Part model, mm, in its own coordinate system. A direction names the side the tool comes from. Coordinates: 2 decimals unless noted, no trailing zeros. Write each loop counter-clockwise with the first axis right and the second up, starting at its lowest first coordinate (ties: lowest second). Pieces come first, ordered by that corner, then holes. Notation, with made-up numbers: (-2.75, 31.5) -> (51.25, 31.5) arc R35 cw to (51.25, 64.5) -> close; hole circle Ø8 at (28.5, -21). An arc over 180 degrees is marked (long way). One line per question, with ' | ' between items. Start each with the question number.
Item 1: Saw through at B-B (y = 0.5). List the corners of the cut face in (x, z), and give its area (3 significant figures).
Item 2: Saw through at C-C (x = -6.25). List the corners of the cut face in (y, z), and give its area (3 significant figures).
Item 3: 3-axis set-ups, long thin cutter, end or side, ignore diameter. For faces 1 (the flat face through (4.7, 0, 14)), 2 (the flat face through (13.178, 0, -8)), 3 (the flat face through (-4.7, 0, 28)), 4 (the flat face through (3, 0, 32)): which of +Z, -Z, +X, -X, +Y, -Y reach the whole face in a straight line?
Item 4: Pin check, flat tips, straight feed: pin 1 (2.5 mm diameter, centred on x = -10.5, y = 1, fed in from +Z); pin 2 (3 mm diameter, centred on y = 2.5, z = 35.5, fed in from -X); pin 3 (1.3 mm diameter, centred on y = -0.5, z = 43.5, fed in from +X). Stop position of each tip, or through.
Item 5: Probe probe 1 along Y at (x, z) = (5.25, 3); probe 2 along Z at (x, y) = (6, 0.75); probe 3 along Z at (x, y) = (9.25, 2.5). List the from-to ranges inside material, lowest first. Write a range as [from, to].
Item 6: Saw through at D-D (z = 39). List the corners of the cut face in (x, y), and give its area (3 significant figures).
Item 7: Saw through at A-A (z = 16.5). List the corners of the cut face in (x, y), and give its area (3 significant figures).
from build123d import *

# Parameters (mm, degrees)
SZKIC1_W                    = 9.4
SZKIC1_H                    = 4.5
DODANIE_WYCI_GNI_CIE1_DEPTH = 51
SZKIC2_W                    = 2.7
SZKIC2_H                    = 9
SZKIC2_W_2                  = 5.3
WYTNIJ_WYCI_GNI_CIE1_DEPTH  = 10
SZKIC4_W                    = 15
SZKIC4_H                    = 10
SZKIC4_W_2                  = 26.356233294
SZKIC4_H_2                  = 5
DODANIE_WYCI_GNI_CIE2_DEPTH = 5
ZAOKR_GLENIE1_R             = 2


with BuildPart() as part:
    # Szkic1 → Dodanie-wyciągnięcie1 (new body)
    with BuildSketch(Plane.XY):
        Polygon((0, 6.95), (4.7, 2.25), (-4.7, 2.25), align=None)
        Rectangle(SZKIC1_W, SZKIC1_H)
    extrude(amount=DODANIE_WYCI_GNI_CIE1_DEPTH)

    # Szkic2 → Wytnij-wyciągnięcie1 (cut)
    with BuildSketch(Plane.XZ.offset(2.25)):
        with Locations((3.35, 27.5)):
            Rectangle(SZKIC2_W, SZKIC2_H)
        with Locations((7.35, 27.5)):
            Rectangle(SZKIC2_W_2, SZKIC2_H)
    extrude(amount=-WYTNIJ_WYCI_GNI_CIE1_DEPTH, mode=Mode.SUBTRACT)

    # Szkic4 → Dodanie-wyciągnięcie2 (add)
    with BuildSketch(Plane.XZ.offset(2.25)):
        Rectangle(SZKIC4_W, SZKIC4_H)
        with Locations((0, -7.5)):
            Rectangle(SZKIC4_W_2, SZKIC4_H_2)
    extrude(amount=-DODANIE_WYCI_GNI_CIE2_DEPTH)

    # Zaokrąglenie1
    zaokr_glenie1_edges = [part.edges().sort_by_distance(p)[0] for p in [
        (4.7, 2.25, 14),
        (-4.7, 2.25, 28),
        (0, 6.95, 25.5),
    ]]
    fillet(zaokr_glenie1_edges, radius=ZAOKR_GLENIE1_R)


solid = part.part
From the geometry:
1) outline: (-13.18, -10) -> (13.18, -10) -> (13.18, -5) -> (7.5, -5) -> (7.5, 5) -> (4.7, 5) -> (4.7, 23) -> (2, 23) -> (2, 32) -> (4.7, 32) -> (4.7, 51) -> (-4.7, 51) -> (-4.7, 5) -> (-7.5, 5) -> (-7.5, -5) -> (-13.18, -5) -> close | area: 690 mm2
2) outline: (-2.25, -10) -> (2.75, -10) -> (2.75, 5) -> (-2.25, 5) -> close | area: 75.0 mm2
3) face 1: +Z, +X, +Y, -Y | face 2: +Z, -Z, +X, +Y, -Y | face 3: +Z, -X, +Y, -Y | face 4: +X, +Y, -Y
4) pin 1: z = -5 | pin 2: x = -4.7 | pin 3: x = 4.7
5) probe 1: [-2.25, 2.75] | probe 2: [-10, 5] | probe 3: [-10, -5]
6) outline: (-4.7, -2.25) -> (4.7, -2.25) -> (4.7, 2.25) -> (1.41, 5.54) arc R2 ccw to (-1.41, 5.54) -> (-4.11, 2.84) arc R2 ccw to (-4.7, 1.42) -> close | area: 63.4 mm2
7) outline: (-4.7, -2.25) -> (4.7, -2.25) -> (4.7, 1.42) arc R2 ccw to (4.11, 2.84) -> (1.41, 5.54) arc R2 ccw to (-1.41, 5.54) -> (-4.11, 2.84) arc R2 ccw to (-4.7, 1.42) -> close | area: 63.4 mm2
